Model file for the job. Use its own axes, mm. A direction names the side the tool comes from. Coordinates: 2 decimals unless noted, no trailing zeros. Write each loop counter-clockwise with the first axis right and the second up, starting at its lowest first coordinate (ties: lowest second). Pieces come first, ordered by that corner, then holes. Notation, with made-up numbers: (66, 61.5) -> (105, 61.5) arc R14 cw to (105, 77.5) -> close; hole circle Ø6 at (73.25, 55.25). An arc over 180 degrees is marked (long way). Answer as a JSON object with one key per item and string values. Group by question number.
from build123d import *

# Parameters (mm, degrees)
CROQUIS1_R              = 9.5
CROQUIS1_R_2            = 10
CROQUIS1_R_3            = 6
SALIENTE_EXTRUIR1_DEPTH = 12
CROQUIS2_R              = 2.144956207
CORTAR_EXTRUIR1_DEPTH   = 3
REDONDEO1_R             = 15
REDONDEO2_R             = 15
CROQUIS4_R              = 16
CORTAR_EXTRUIR2_DEPTH   = 8


with BuildPart() as part:
    # Croquis1 → Saliente-Extruir1 (new body)
    with BuildSketch(Plane.XY):
        with BuildLine():
            Line((380, -45.4), (380, -25.4))
            Line((380, -25.4), (-25.4, -25.4))
            Line((-25.4, -25.4), (-25.4, 25.4))
            Line((-25.4, 25.4), (457.4, 25.4))
            Line((457.4, 25.4), (457.4, -25.4))
            Line((457.4, -25.4), (420, -25.4))
            Line((420, -25.4), (420, -45.4))
            ThreePointArc((420, -45.4), (400, -65.4), (380, -45.4))
        make_face()
        with Locations((432, 0)):
            Circle(CROQUIS1_R, mode=Mode.SUBTRACT)
        with Locations((40, 0)):
            Circle(CROQUIS1_R_2, mode=Mode.SUBTRACT)
        with Locations((312, 0)):
            Circle(CROQUIS1_R_3, mode=Mode.SUBTRACT)
        with Locations((400, -45.4)):
            Circle(CROQUIS1_R_2, mode=Mode.SUBTRACT)
        with BuildLine():
            Line((-6.28, -7.782133384), (-6.28, 7.782133384))
            ThreePointArc((-6.28, 7.782133384), (0, 10), (6.28, 7.782133384))
            Line((6.28, 7.782133384), (6.28, -7.782133384))
            ThreePointArc((6.28, -7.782133384), (0, -10), (-6.28, -7.782133384))
        make_face(mode=Mode.SUBTRACT)
    extrude(amount=SALIENTE_EXTRUIR1_DEPTH)

    # Croquis2 → Cortar-Extruir1 (cut)
    with BuildSketch(Plane(origin=(0, 0, 0), x_dir=(-1, 0, 0), z_dir=(0, 0, -1))):
        with Locations((-66.437001332, -11.298220954)):
            Circle(CROQUIS2_R)
    extrude(amount=-CORTAR_EXTRUIR1_DEPTH, mode=Mode.SUBTRACT)

    # Redondeo1
    redondeo1_edges = [part.edges().sort_by_distance(p)[0] for p in [
        (-25.4, 25.4, 6),
        (-25.4, -25.4, 6),
    ]]
    fillet(redondeo1_edges, radius=REDONDEO1_R)

    # Redondeo2
    redondeo2_edges = [part.edges().sort_by_distance(p)[0] for p in [
        (457.4, 25.4, 6),
        (457.4, -25.4, 6),
    ]]
    fillet(redondeo2_edges, radius=REDONDEO2_R)

    # Croquis4 → Cortar-Extruir2 (cut)
    with BuildSketch(Plane.XY.offset(12)):
        with Locations((40, 0)):
            Circle(CROQUIS4_R)
    extrude(amount=-CORTAR_EXTRUIR2_DEPTH, mode=Mode.SUBTRACT)


solid = part.part
(1) Cut at C-C on z = 7.75. List the corners of the cut face in (x, y).
(2) Cut at D-D on x = 40. List the corners of the cut face in (y, z).
(3) Cut at B-B on y = 0. List the corners of the cut face in (x, z), plus the area to 3 significant figures.
(4) Wall check: probe 1 along Y at (x, z) = (400, 8); probe 2 along Y at (x, z) = (312, 7.25); probe 3 along Y at (x, z) = (378, 2.25). Give the ranges that are in metal, low to high.
(5) Pin check, flat tips, straight feed: pin 1 (1 mm diameter, centred on y = -32, z = 7.5, fed in from +X); pin 2 (6 mm diameter, centred on x = 430.5, z = 7.5, fed in from -Y); pin 3 (2 mm diameter, centred on y = -13, z = 10.5, fed in from -X). Stop position of each tip, or through.
(6) Pull direction X, two halves, no side cores. Call faces 4 (the face through (219, 1, 12)), 5 (the face through (-6.28, 0, 6)), 6 (the face through (440.776, -3.639, 5.916)), 7 (the face through (-25.4, 0, 6)): released by +X, released by -X, zero draft, split by the parting line, or undercut.
(7) Cut at A-A on x = 432. List the corners of the cut face in (y, z), plus the area to 3 significant figures.
(8) 3-axis set-ups, long thin cutter, end or side, ignore diameter. For faces 1 (the face through (24.015, 0.703, 8.056)), 2 (the face through (0, 10, 6)), 3 (the face through (420, -35, 6)): which of +Z, -Z, +X, -X, +Y, -Y reach the whole face in a straight line?
Results found:
{
 "1": {"outline": "(-25.4, -10.4) arc R15 ccw to (-10.4, -25.4) -> (380, -25.4) -> (380, -45.4) arc R20 ccw to (420, -45.4) -> (420, -25.4) -> (442.4, -25.4) arc R15 ccw to (457.4, -10.4) -> (457.4, 10.4) arc R15 ccw to (442.4, 25.4) -> (-10.4, 25.4) arc R15 ccw to (-25.4, 10.4) -> close; hole (-6.28, -7.78) arc R10 ccw to (6.28, -7.78) -> (6.28, 7.78) arc R10 ccw to (-6.28, 7.78) -> close; hole circle Ø32 at (40, 0); hole circle Ø12 at (312, 0); hole circle Ø20 at (400, -45.4); hole circle Ø19 at (432, 0)"},
 "2": {"outline": "(-25.4, 0) -> (-10, 0) -> (-10, 4) -> (-16, 4) -> (-16, 12) -> (-25.4, 12) -> close; (10, 0) -> (25.4, 0) -> (25.4, 12) -> (16, 12) -> (16, 4) -> (10, 4) -> close"},
 "3": {"outline": "(-25.4, 0) -> (-6.28, 0) -> (-6.28, 12) -> (-25.4, 12) -> close; (6.28, 0) -> (30, 0) -> (30, 4) -> (24, 4) -> (24, 12) -> (6.28, 12) -> close; (50, 0) -> (306, 0) -> (306, 12) -> (56, 12) -> (56, 4) -> (50, 4) -> close; (318, 0) -> (422.5, 0) -> (422.5, 12) -> (318, 12) -> close; (441.5, 0) -> (457.4, 0) -> (457.4, 12) -> (441.5, 12) -> close", "area": "4,930 mm²"},
 "4": {"probe 1": "y = -65.4 to -55.4, -35.4 to 25.4", "probe 2": "y = -25.4 to -6, 6 to 25.4", "probe 3": "y = -25.4 to 25.4"},
 "5": {"pin 1": "stops at x = 420", "pin 2": "stops at y = -25.4", "pin 3": "stops at x = -25.31"},
 "6": {"face 4": "zero draft", "face 5": "undercut", "face 6": "undercut", "face 7": "released by -X"},
 "7": {"outline": "(-25.4, 0) -> (-9.5, 0) -> (-9.5, 12) -> (-25.4, 12) -> close; (9.5, 0) -> (25.4, 0) -> (25.4, 12) -> (9.5, 12) -> close", "area": "382 mm²"},
 "8": {"face 1": "+Z", "face 2": "+Z, -Z", "face 3": "+Z, -Z, +X, -Y"}
}
